```python
from build123d import *

# Parameters (mm, degrees)
F0_W        = 2.9410525192
F0_H        = 2.54
F1_DEPTH    = 38.1
F2_T1_DEPTH = 68.2618004135
F3_R        = 5.08
F4_T1_DEPTH = 23.6793240582


# Not quite as in the source:
# - a fillet or chamfer that OpenCascade refuses, or shapes differently, is made with other operations: its cross-section is extruded or revolved along the edge and cut away or added


with BuildPart() as f1:
    # F0 (on Top) → F1 (new body)
    with BuildSketch(Plane.XY):
        with Locations((-36.622652784, 43.036242947)):
            Rectangle(F0_W, F0_H)
    extrude(amount=F1_DEPTH)

    # F2: chamfer of 12.7 on 1 edges, made by hand

    # F2_s2 → F2_t1 (cut)
    with BuildSketch(Plane.YZ.offset(-70.7535529908)):
        Polygon((41.766242947, 25.4), (54.466242947, 38.1), (41.766242947, 38.1), align=None)
    extrude(amount=F2_T1_DEPTH, mode=Mode.SUBTRACT)

    # F3
    f3_edges = [f1.edges().sort_by_distance(p)[0] for p in [
        (-36.622653, 41.766243, 25.4),
    ]]
    fillet(f3_edges, radius=F3_R)

    # F4: fillet of radius 5.08 on 1 edges, made by hand

    # F4_s2 → F4_t1 (cut)
    with BuildSketch(Plane.YZ.offset(-48.4623148131)):
        with BuildLine():
            ThreePointArc((43.2541404986, 26.8878975516), (44.0360308613, 25.4270750946), (44.306242947, 23.7923456922))
            Line((44.306242947, 23.7923456922), (44.306242947, 27.94))
            Line((44.306242947, 27.94), (43.2541404986, 26.8878975516))
        make_face()
    extrude(amount=F4_T1_DEPTH, mode=Mode.SUBTRACT)


solid = f1.part
```
Geometry check sheet. Reference: the model listing, model coordinates, mm. Coordinates: 2 decimals unless noted, no trailing zeros. Order: outer loops, then holes, each group sorted by start corner. A loop starts at its lowest first (then second) coordinate and runs counter-clockwise, first axis right, second up. Notation, with made-up numbers: M 1.5,65.25 L 41.5,65.25 A12 ccw 41.5,86.25 Z; hole C 65.25,54 d6. An arc over 180 degrees is marked long. Answer as a JSON object with one key per item and string values.
Q1. Cross-section at B-B on y = 43.65. Record the cut outline in (x, z).
Results are:
{"outline": "M -38.09,0 L -35.15,0 L -35.15,26.29 L -38.09,26.29 Z"}
Q2. Release check for a two-part mould opening along Z. For faces 1 (the cylindrical face through (-36.64, 44.03, 25.45)), 2 (the flat face through (-37, 43, 0)), 3 (the flat face through (-38.093, 43, 13)) record: released by +Z, released by -Z, zero draft, split by the parting line, or undercut.
Results are:
{"face 1": "released by +Z", "face 2": "released by -Z", "face 3": "zero draft"}
Q3. Cross-section at C-C on y = 42.6. Record the cut outline in (x, z), and give its area (3 significant figures).
Results are:
{"outline": "M -38.09,0 L -35.15,0 L -35.15,26.08 L -38.09,26.08 Z", "area": "76.7 mm²"}
Q4. Scan lines: line 1 (Z direction, x = -36.05, y = 42.5); line 2 (Z direction, x = -35.9, y = 43.15). Record each from-to range of solid material in increasing order.
Results are:
{"line 1": "z = 0 to 25.93", "line 2": "z = 0 to 26.78"}
Q5. Cross-section at A-A on x = -37. Record the cut outline in (y, z), and give its area (3 significant figures).
Results are:
{"outline": "M 41.77,0 L 44.31,0 L 44.31,23.79 A5.08 ccw 43.25,26.89 A5.08 ccw 41.77,23.3 Z", "area": "65.6 mm²"}
